from build123d import *
from build123d.topology import SkipClean

# Parameters (mm, degrees)
SKETCH1_R                                          = 14.2875
BOSS_EXTRUDE1_DEPTH                                = 3.175
F_6_CLEARANCE_HOLE3_D                              = 4.3053
CUT_EXTRUDE1_DEPTH                                 = 255.792513626
CHAMFER1_SIZE                                      = 3.81
SKETCH10_W                                         = 50.8
SKETCH10_H                                         = 38.1
BOSS_EXTRUDE2_DEPTH                                = 6.35
CHAMFER2_SIZE                                      = 3.175
CSK_FOR_10_FLAT_HEAD_MACHINE_SCREW_100_D           = 5.6134
CSK_FOR_10_FLAT_HEAD_MACHINE_SCREW_100_CSINK_D     = 9.779
CSK_FOR_10_FLAT_HEAD_MACHINE_SCREW_100_CSINK_ANGLE = 100
F_1_4_0_25_DIAMETER_HOLE1_D                        = 6.35
CSK_FOR_6_FLAT_HEAD_MACHINE_SCREW_100_D            = 4.3053
CSK_FOR_6_FLAT_HEAD_MACHINE_SCREW_100_CSINK_D      = 7.0866
CSK_FOR_6_FLAT_HEAD_MACHINE_SCREW_100_CSINK_ANGLE  = 100
F_15_32_0_46875_DIAMETER_HOLE1_D                   = 11.90625


# Read off the part's stored shape, not the designer's step: DeleteFace1
with BuildPart() as part:
    # Sketch1 → Boss-Extrude1 (new, symmetric)
    with BuildSketch(Plane.XY):
        Polygon((0, 19.05), (-28.575, 19.05), (-28.575, -19.05), (0, -19.05), (247.281942035, -19.05), (254, 19.05), align=None)
        Circle(SKETCH1_R, mode=Mode.SUBTRACT)
    extrude(amount=BOSS_EXTRUDE1_DEPTH, both=True)

    # #6 Clearance Hole3 (through all)
    with Locations(Plane.XY.offset(3.175)):
        with Locations((229.388701471, 8.923791784), (229.282371239, -11.346798968), (203.503161764, -11.143926969), (203.608782335, 8.991375351), (165.672159691, 8.991375351), (165.672159691, -11.143926969), (151.067159691, 0)):
            Hole(F_6_CLEARANCE_HOLE3_D / 2)

    # Sketch9 → Cut-Extrude1 (cut, through all)
    with BuildSketch(Plane.XY.offset(3.175)):
        Polygon((254, 19.05), (247.281942035, -19.05), (237.352085197, -19.05), (237.352085197, 19.05), align=None)
    extrude(amount=-CUT_EXTRUDE1_DEPTH, mode=Mode.SUBTRACT)

    # Chamfer1
    chamfer1_edges = [part.edges().sort_by_distance(p)[0] for p in [
        (-28.575, -19.05, 0),
        (-28.575, 19.05, 0),
        (237.352085197, 19.05, 0),
        (237.352085197, -19.05, 0),
    ]]
    chamfer(chamfer1_edges, length=CHAMFER1_SIZE)

    # Sketch10 → Boss-Extrude2 (add, through all)
    with BuildSketch(Plane.XY.offset(3.175)):
        with Locations((-50.165, 0)):
            Rectangle(SKETCH10_W, SKETCH10_H)
    extrude(amount=-BOSS_EXTRUDE2_DEPTH)

    # Chamfer2
    chamfer2_edges = [part.edges().sort_by_distance(p)[0] for p in [
        (-75.565, -19.05, 0),
        (-75.565, 19.05, 0),
    ]]
    chamfer(chamfer2_edges, length=CHAMFER2_SIZE)

    # CSK for #10 Flat Head Machine Screw (100)1 (through all)
    with Locations(Plane.XY.offset(3.175)):
        with Locations((-65.405, 0)):
            CounterSinkHole(CSK_FOR_10_FLAT_HEAD_MACHINE_SCREW_100_D / 2, CSK_FOR_10_FLAT_HEAD_MACHINE_SCREW_100_CSINK_D / 2, counter_sink_angle=CSK_FOR_10_FLAT_HEAD_MACHINE_SCREW_100_CSINK_ANGLE)

    # 1/4 (0.25) Diameter Hole1 (through all)
    with Locations(Plane.XY.offset(3.175)):
        with Locations((-33.655, 0)):
            Hole(F_1_4_0_25_DIAMETER_HOLE1_D / 2)

    # CSK for #6 Flat Head Machine Screw (100)1 (through all)
    with Locations(Plane(origin=(0, 0, -3.175), x_dir=(-1, 0, 0), z_dir=(0, 0, -1))):
        with Locations((-151.067159691, 0), (-165.672159691, -11.143926969), (-165.672159691, 8.991375351)):
            CounterSinkHole(CSK_FOR_6_FLAT_HEAD_MACHINE_SCREW_100_D / 2, CSK_FOR_6_FLAT_HEAD_MACHINE_SCREW_100_CSINK_D / 2, counter_sink_angle=CSK_FOR_6_FLAT_HEAD_MACHINE_SCREW_100_CSINK_ANGLE)

    # 15/32 (0.46875) Diameter Hole1 (through all)
    with Locations(Plane(origin=(0, 0, -3.175), x_dir=(-1, 0, 0), z_dir=(0, 0, -1))):
        with Locations((-93.967218212, 0)):
            Hole(F_15_32_0_46875_DIAMETER_HOLE1_D / 2)

    # DeleteFace1 outline → DeleteFace1 (revolve)
    with SkipClean():  # the faces are left unmerged after this step: merging them gives an invalid solid
        with BuildSketch(Plane(origin=(-65.405, 0, 0), x_dir=(1, 0, 0), z_dir=(0, -1, 0))):
            Polygon((2.8067, 3.175), (2.8067, 1.427323288), (4.8895, 3.175), align=None)
        revolve(axis=Axis((-65.405, 0, 0), (0, 0, 1)))
    add(part.part.scale(1), mode=Mode.REPLACE)  # the faces are merged on a copy

    # DeleteFace1 2 outline → DeleteFace1 2 (revolve)
    with BuildSketch(Plane(origin=(165.672159691, 8.991375351, 0), x_dir=(1, 0, 0), z_dir=(0, -1, 0))):
        Polygon((3.5433, -3.175), (2.15265, -2.008106098), (2.15265, -3.175), align=None)
    revolve(axis=Axis((165.672159691, 8.991375351, 0), (0, 0, 1)))

    # DeleteFace1 3 outline → DeleteFace1 3 (revolve)
    with BuildSketch(Plane(origin=(165.672159691, -11.143926969, 0), x_dir=(1, 0, 0), z_dir=(0, -1, 0))):
        Polygon((3.5433, -3.175), (2.15265, -2.008106098), (2.15265, -3.175), align=None)
    revolve(axis=Axis((165.672159691, -11.143926969, 0), (0, 0, 1)))

    # DeleteFace1 4 outline → DeleteFace1 4 (revolve)
    with BuildSketch(Plane(origin=(151.067159691, 0, 0), x_dir=(1, 0, 0), z_dir=(0, -1, 0))):
        Polygon((3.5433, -3.175), (2.15265, -2.008106098), (2.15265, -3.175), align=None)
    revolve(axis=Axis((151.067159691, 0, 0), (0, 0, 1)))


solid = part.part
Geometry check sheet. Reference: the model listing, model coordinates, mm. Give positions to 0.01 mm unless a question says otherwise; leave off trailing zeros. Write each loop counter-clockwise with the first axis right and the second up, starting at its lowest first coordinate (ties: lowest second). Pieces come first, ordered by that corner, then holes. Notation, with made-up numbers: M 56.25,-27.5 L 114.25,-27.5 A14 cw 114.25,-8.5 Z; hole C 69.25,-1 d8. An arc over 180 degrees is marked long. One line per question, with ' | ' between items.
1. Mould release check, pull along Y, two halves, no side actions. Record for faces 1 (the face through (88.02, 0.26, 0.04)), 2 (the face through (78, -19.05, 0)), 3 (the face through (-14.274, 0.628, -0.044)), 4 (the face through (-75.565, 0, 0)): released by +Y, released by -Y, zero draft, split by the parting line, or undercut.
Ans:
face 1: undercut | face 2: released by -Y | face 3: undercut | face 4: zero draft
2. Scan lines: line 1 along X through (y, z) = (-1.5, 1.5) (3 decimals); line 2 along Y through (x, z) = (94, 1.5); line 3 along X through (y, z) = (-2.5, -2.5) (3 decimals). Record each from-to range of solid material in increasing order. Write a range as from..to.
Ans:
line 1: -75.565..-67.777, -63.033..-36.453, -30.857..-14.209, 14.209..88.206, 99.728..149.523, 152.611..237.352 | line 2: -19.05..-5.95, 5.95..19.05 | line 3: -75.565..-66.681, -64.129..-35.612, -31.698..-14.067, 14.067..88.564, 99.37..237.352
3. Cross-section at B-B (x = 97). Enter the section's corners in (y, z) (3 decimals).
Ans:
outline: M -19.05,-3.175 L -5.123,-3.175 L -5.123,3.175 L -19.05,3.175 Z; M 5.123,-3.175 L 19.05,-3.175 L 19.05,3.175 L 5.123,3.175 Z
